from build123d import *

# Parameters (mm, degrees)
SCHIZZO1_W                            = 85
SCHIZZO1_H                            = 72
ESTRUSIONE_ESTRUSIONE1_DEPTH          = 2
RACCORDO1_R                           = 4
RACCORDO3_R                           = 2
RACCORDO4_R                           = 2
RACCORDO5_R                           = 2
RACCORDO6_R                           = 2
TAGLIO_ESTRUSIONE1_REACH              = 62.453
SCHIZZO2_W                            = 39.2
SCHIZZO2_H                            = 10
SCHIZZO2_W_2                          = 26.2
FORO_SVASATO_PER_VITE_M3_1_AT_2_COUNT = 2
FORO_SVASATO_PER_VITE_M3_1_AT_2_PITCH = 65.075876997
FORO_SVASATO_PER_VITE_M3_1_AT_3_COUNT = 2
FORO_SVASATO_PER_VITE_M3_1_AT_3_PITCH = 100.816019396
FORO_SVASATO_PER_VITE_M3_1_AT_4_COUNT = 2
FORO_SVASATO_PER_VITE_M3_1_AT_4_PITCH = 77


with BuildPart() as part:
    # Schizzo1 → Estrusione-Estrusione1 (new body)
    with BuildSketch(Plane.XY):
        Rectangle(SCHIZZO1_W, SCHIZZO1_H)
        Polygon((0, 43), (42.5, 36), (-42.5, 36), align=None)
    extrude(amount=ESTRUSIONE_ESTRUSIONE1_DEPTH)

    # Raccordo1
    raccordo1_edges = [part.edges().sort_by_distance(p)[0] for p in [
        (0, 43, 1),
    ]]
    fillet(raccordo1_edges, radius=RACCORDO1_R)

    # Raccordo3
    raccordo3_edges = [part.edges().sort_by_distance(p)[0] for p in [
        (42.5, 36, 1),
    ]]
    fillet(raccordo3_edges, radius=RACCORDO3_R)

    # Raccordo4
    raccordo4_edges = [part.edges().sort_by_distance(p)[0] for p in [
        (42.5, -36, 1),
    ]]
    fillet(raccordo4_edges, radius=RACCORDO4_R)

    # Raccordo5
    raccordo5_edges = [part.edges().sort_by_distance(p)[0] for p in [
        (-42.5, -36, 1),
    ]]
    fillet(raccordo5_edges, radius=RACCORDO5_R)

    # Raccordo6
    raccordo6_edges = [part.edges().sort_by_distance(p)[0] for p in [
        (-42.5, 36, 1),
    ]]
    fillet(raccordo6_edges, radius=RACCORDO6_R)

    # Schizzo2 → Taglio-Estrusione1 (cut, up to next)
    with BuildSketch(Plane.XY.offset(2), mode=Mode.PRIVATE) as taglio_estrusione1_sk1:
        with Locations((7.5, -11.99)):
            Rectangle(SCHIZZO2_W, SCHIZZO2_H)
    taglio_estrusione1_tool1 = extrude(taglio_estrusione1_sk1.sketch, amount=-TAGLIO_ESTRUSIONE1_REACH, mode=Mode.PRIVATE) & part.part
    # Schizzo2 → Taglio-Estrusione1 (cut, up to next)
    with BuildSketch(Plane.XY.offset(2), mode=Mode.PRIVATE) as taglio_estrusione1_sk2:
        with Locations((7, -26)):
            Rectangle(SCHIZZO2_W_2, SCHIZZO2_H)
    taglio_estrusione1_tool2 = extrude(taglio_estrusione1_sk2.sketch, amount=-TAGLIO_ESTRUSIONE1_REACH, mode=Mode.PRIVATE) & part.part
    add(taglio_estrusione1_tool1.solids().sort_by_distance((7.5, -11.99, 2))[0], mode=Mode.SUBTRACT)
    add(taglio_estrusione1_tool2.solids().sort_by_distance((7, -26, 2))[0], mode=Mode.SUBTRACT)

    # Schizzo4 → Foro svasato per Vite M3-1 (revolve, cut)
    with BuildSketch(Plane(origin=(-38.5, 33.075876997, 2), x_dir=(0, -1, 0), z_dir=(1, 0, 0))):
        Polygon((0, 0), (0, 2), (1.7, 2), (1.7, 1.45), (3.15, 0), align=None)
    foro_svasato_per_vite_m3_1 = revolve(axis=Axis((-38.5, 33.075876997, 8.35), (0, 0, -1)), mode=Mode.SUBTRACT)

    # Foro svasato per Vite M3-1 at 2: Foro svasato per Vite M3-1 ×2
    with Locations(*[(0, -i * FORO_SVASATO_PER_VITE_M3_1_AT_2_PITCH, 0) for i in range(1, FORO_SVASATO_PER_VITE_M3_1_AT_2_COUNT)]):
        add(foro_svasato_per_vite_m3_1, mode=Mode.SUBTRACT)

    # Foro svasato per Vite M3-1 at 3: Foro svasato per Vite M3-1 ×2
    with Locations(*[Vector(0.7637675089853256, -0.6454914346591678, 0) * (i * FORO_SVASATO_PER_VITE_M3_1_AT_3_PITCH) for i in range(1, FORO_SVASATO_PER_VITE_M3_1_AT_3_COUNT)]):
        add(foro_svasato_per_vite_m3_1, mode=Mode.SUBTRACT)

    # Foro svasato per Vite M3-1 at 4: Foro svasato per Vite M3-1 ×2
    with Locations(*[(i * FORO_SVASATO_PER_VITE_M3_1_AT_4_PITCH, 0, 0) for i in range(1, FORO_SVASATO_PER_VITE_M3_1_AT_4_COUNT)]):
        add(foro_svasato_per_vite_m3_1, mode=Mode.SUBTRACT)


solid = part.part
Could you check a few things on this model? Use its own coordinates, in mm. A direction names the side the tool comes from. Give positions to 0.01 mm unless a question says otherwise; leave off trailing zeros. Loops run counter-clockwise (first coordinate to the right, second up) from the corner with the lowest first, then second, coordinate; pieces in that order, holes last. Notation, with made-up numbers: (71, 88) -> (114, 88) arc R13 ccw to (114, 109) -> close; hole circle Ø6 at (-30.75, 31.25). An arc over 180 degrees is marked (long way). Return JSON: item names as keys, results as strings.
Item 1: Which directions (+Z, -Z, +X, -X, +Y, -Y) give clear straight access to the entire face, cutting with the end or side of a thin tool? Please do faces 1 (the flat face through (7, -6.99, 1)), 2 (the flat face through (42.5, 0, 1)).
Geometry results:
{"face 1": "+Z, -Z", "face 2": "+Z, -Z, +X, +Y, -Y"}
Item 2: If we section it at A-A on y = -32: List the corners of the cut face in (x, z) for me, plus the area to 3 significant figures.
Geometry results:
{"outline": "(-42.5, 0) -> (-40.2, 0) -> (-40.2, 0.55) -> (-41.65, 2) -> (-42.5, 2) -> close; (-36.8, 0) -> (36.8, 0) -> (36.8, 0.55) -> (35.35, 2) -> (-35.35, 2) -> (-36.8, 0.55) -> close; (40.2, 0) -> (42.5, 0) -> (42.5, 2) -> (41.65, 2) -> (40.2, 0.55) -> close", "area": "152 mm²"}
Item 3: I need wall thicknesses on L1, parallel to X at y = -32, z = 0.4; L2, parallel to Y at x = 39.5, z = 0.15; L3, parallel to Y at x = 3.5, z = 0.9. Which ranges of each line are inside material? Lowest first, please. Write a range as from..to.
Geometry results:
{"L1": "x = -42.5..-40.2, -36.8..36.8, 40.2..42.5", "L2": "y = -36..-33.37, -30.63..31.7, 34.45..36.49", "L3": "y = -36..-31, -21..-16.99, -6.99..42.42"}
Item 4: If we section it at D-D on x = -38.5: List the corners of the cut face in (y, z) for me.
Geometry results:
{"outline": "(-36, 0) -> (-33.7, 0) -> (-33.7, 0.55) -> (-35.15, 2) -> (-36, 2) -> close; (-30.3, 0) -> (31.38, 0) -> (31.38, 0.55) -> (29.93, 2) -> (-28.85, 2) -> (-30.3, 0.55) -> close; (34.78, 0) -> (36.66, 0) -> (36.66, 2) -> (36.23, 2) -> (34.78, 0.55) -> close"}
Item 5: We'd pull the mould along Y, two halves only. Please class faces 3 (the cylindrical face through (41.93, -35.4, 1.01)), 4 (the cylindrical face through (-42.04, 35.58, 1.01)), 5 (the flat face through (-6.1, -26, 1)): +Y half, -Y half, draft (parallel to the pull), parting line (faces both ways), or undercut.
Geometry results:
{"face 3": "-Y half", "face 4": "+Y half", "face 5": "undercut"}
Item 6: I'm going to push flat-ended pins straight in: pin 1 (4.5 mm diameter, centred on x = 38.5, y = -32, fed in from +Z); pin 2 (0.6 mm diameter, centred on x = -1, z = 0.5, fed in from +Y); pin 3 (10 mm diameter, centred on x = 17, y = -25.5, fed in from -Z). Where does each tip first touch, or does it pass through?
Geometry results:
{"pin 1": "stops at z = 1.1", "pin 2": "stops at y = 42.88", "pin 3": "stops at z = 0"}
Item 7: If we section it at C-C on y = -9: List the corners of the cut face in (x, z) for me.
Geometry results:
{"outline": "(-42.5, 0) -> (-12.1, 0) -> (-12.1, 2) -> (-42.5, 2) -> close; (27.1, 0) -> (42.5, 0) -> (42.5, 2) -> (27.1, 2) -> close"}
Item 8: If we section it at B-B on x = -11: List the corners of the cut face in (y, z) for me.
Geometry results:
{"outline": "(-36, 0) -> (-16.99, 0) -> (-16.99, 2) -> (-36, 2) -> close; (-6.99, 0) -> (41.19, 0) -> (41.19, 2) -> (-6.99, 2) -> close"}
